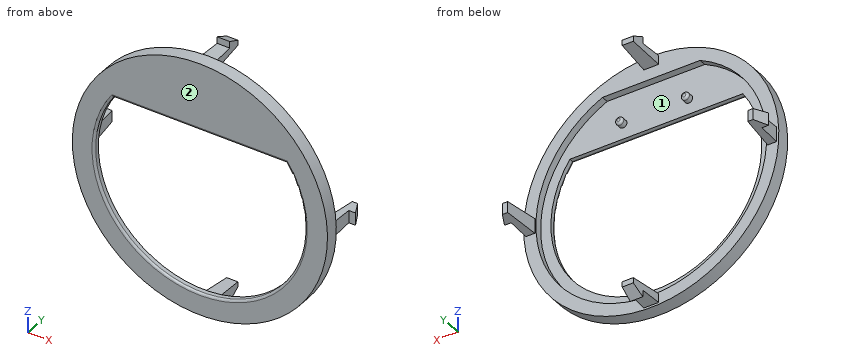
from build123d import *

# Parameters (mm, degrees)
SKETCH1_R           = 14.605
BOSS_EXTRUDE1_DEPTH = 1.524
CUT_EXTRUDE1_DEPTH  = 0.8128
SKETCH4_R           = 0.4445
BOSS_EXTRUDE2_DEPTH = 0.8128
CUT_EXTRUDE2_DEPTH  = 21.670575557
FILLET1_R           = 0.254
FILLET3_R           = 0.254
SNAP_START          = 13.7414
SNAP_HOOK1_DEPTH    = 0.6096
SNAP_START_2        = -0.714869456
SNAP_HOOK1_2_DEPTH  = 1.429738912
SNAP_START_3        = -0.847985215
SNAP_HOOK1_3_DEPTH  = 1.69597043
SNAP_START_4        = 12
SNAP_HOOK1_4_DEPTH  = 4
CIRPATTERN1_COUNT   = 4


with BuildPart() as part:
    # Sketch1 → Boss-Extrude1 (new body)
    with BuildSketch(Plane(origin=(0, 0, 0), x_dir=(1, 0, 0), z_dir=(0, 1, 0))):
        with Locations(Location((0, 0, 0), (0, 0, 270))):
            Circle(SKETCH1_R)
    extrude(amount=BOSS_EXTRUDE1_DEPTH)

    # Sketch3 → Cut-Extrude1 (cut)
    with BuildSketch(Plane(origin=(0, 1.524, 0), x_dir=(1, 0, 0), z_dir=(0, 1, 0))):
        with BuildLine():
            Line((-5.588, -11.967686493), (5.588, -11.967686493))
            ThreePointArc((5.588, -11.967686493), (0, 13.208), (-5.588, -11.967686493))
        make_face()
    extrude(amount=-CUT_EXTRUDE1_DEPTH, mode=Mode.SUBTRACT)

    # Sketch4 → Boss-Extrude2 (add)
    with BuildSketch(Plane(origin=(0, 0.7112, 0), x_dir=(1, 0, 0), z_dir=(0, 1, 0))):
        with Locations(Location((-3.7592, -8.6233, 0), (0, 0, 90))):
            Circle(SKETCH4_R)
        with Locations(Location((3.7592, -8.6233, 0), (0, 0, 90))):
            Circle(SKETCH4_R)
    extrude(amount=BOSS_EXTRUDE2_DEPTH)

    # Sketch5 → Cut-Extrude2 (cut, through all)
    with BuildSketch(Plane(origin=(0, 0.7112, 0), x_dir=(1, 0, 0), z_dir=(0, 1, 0))):
        with BuildLine():
            Line((-9.940854815, -6.887686493), (9.870656967, -6.887686493))
            ThreePointArc((9.870656967, -6.887686493), (-0.035098924, 12.065), (-9.940854815, -6.887686493))
        make_face()
    extrude(amount=-CUT_EXTRUDE2_DEPTH, mode=Mode.SUBTRACT)

    # Fillet1
    fillet1_edges = [part.edges().sort_by_distance(p)[0] for p in [
        (-0.035098924, 0, -12.065),
        (-0.035098924, 0, 6.887686493),
    ]]
    fillet(fillet1_edges, radius=FILLET1_R)

    # Fillet3
    fillet3_edges = [part.edges().sort_by_distance(p)[0] for p in [
        (-3.7592, 1.524, 9.0678),
        (3.7592, 1.524, 9.0678),
    ]]
    fillet(fillet3_edges, radius=FILLET3_R)

    # Snap Hook1: read off the stored shape, not the designer's step
    # Snap Hook1 outline → Snap Hook1 (add)
    with BuildSketch(Plane.XY.offset(SNAP_START)):
        Polygon((-0.847985215, 1.524), (0.847985215, 1.524), (0.635, 5.588), (-0.635, 5.588), align=None)
    snap_hook1 = extrude(amount=SNAP_HOOK1_DEPTH)

    # Snap Hook1 2 outline → Snap Hook1 2 (add)
    with BuildSketch(Plane.YZ.offset(SNAP_START_2)):
        Polygon((1.524, 13.7414), (1.524, 13.335), (5.588, 13.7414), align=None)
        Polygon((4.064, 15.113), (4.064, 14.351), (5.588, 14.351), align=None)
    snap_hook1_2 = extrude(amount=SNAP_HOOK1_2_DEPTH)

    # Snap Hook1 3 outline → Snap Hook1 3 (add)
    with BuildSketch(Plane.YZ.offset(SNAP_START_3)):
        Polygon((1.524, 13.7414), (1.524, 13.335), (5.588, 13.7414), align=None)
    snap_hook1_3 = extrude(amount=SNAP_HOOK1_3_DEPTH)

    # Snap Hook1 4 outline → Snap Hook1 4 (cut)
    with BuildSketch(Plane.XY.offset(SNAP_START_4)):
        Polygon((0.847985215, 1.524), (0.847985215, 7), (0.561000216, 7), (0.635, 5.588), align=None)
        Polygon((-0.635, 5.588), (-0.561000216, 7), (-0.847985215, 7), (-0.847985215, 1.524), align=None)
    snap_hook1_4 = extrude(amount=SNAP_HOOK1_4_DEPTH, mode=Mode.SUBTRACT)

    # CirPattern1: Snap Hook1, Snap Hook1 2, Snap Hook1 3, Snap Hook1 4 ×4 about axis
    cirpattern1_axis = Axis((0, 1.524, 0), (0, 1, 0))
    add([snap_hook1.rotate(cirpattern1_axis, i * 360 / CIRPATTERN1_COUNT) for i in range(1, CIRPATTERN1_COUNT)])
    add([snap_hook1_2.rotate(cirpattern1_axis, i * 360 / CIRPATTERN1_COUNT) for i in range(1, CIRPATTERN1_COUNT)])
    add([snap_hook1_3.rotate(cirpattern1_axis, i * 360 / CIRPATTERN1_COUNT) for i in range(1, CIRPATTERN1_COUNT)])
    add([snap_hook1_4.rotate(cirpattern1_axis, i * 360 / CIRPATTERN1_COUNT) for i in range(1, CIRPATTERN1_COUNT)], mode=Mode.SUBTRACT)


solid = part.part
CAD build for the part. Positions are in the model's coordinates, mm. Face numbers are marked on the shaded views. Round coordinates to 2 decimals unless told otherwise and drop trailing zeros. Order: outer loops, then holes, each group sorted by start corner. A loop starts at its lowest first (then second) coordinate and runs counter-clockwise, first axis right, second up. Notation, with made-up numbers: M 56.25,-18.5 L 100.25,-18.5 A23 ccw 100.25,5.5 Z; hole C 70,31.5 d10. An arc over 180 degrees is marked long. Use one line per item in the form item = value.
Q1. Probe L1, parallel to X at y = 1.25, z = 0 (3 decimals); L2, parallel to X at y = 0.5, z = 0 (3 decimals); L3, parallel to Y at x = 4.5, z = -13. List the from-to ranges inside material, lowest first.
Recorded:
L1 = -14.605 to -13.208, 13.208 to 14.605
L2 = -14.605 to -12.1, 12.03 to 14.605
L3 = 0 to 1.52
Q2. Saw through at B-B on z = 10. Give the cut face in (x, y), then the cut area to 3 significant figures.
Recorded:
outline = M -10.64,0 L 10.64,0 L 10.64,1.52 L 8.63,1.52 L 8.63,0.71 L -8.63,0.71 L -8.63,1.52 L -10.64,1.52 Z
area = 18.4 mm^2
Q3. Flat gauge pins, fed straight in: P1, Ø1.4, axis at x = 0.5, y = 3, coming from the -Z side; P2, Ø0.9, axis at x = -1, y = 1, coming from the -Z side; P3, Ø1.5, axis at x = -5, z = -11.5, coming from the +Y side; P4, Ø12, axis at x = 8.5, z = 6, coming from the -Y side. Where does each tip first touch, or does it go through?
Recorded:
P1 = -14.35
P2 = -14.59
P3 = 1.52
P4 = 0
Q4. Saw through at A-A on y = 4.9. Give the cut face in (x, z) (3 decimals).
Recorded:
outline = M -14.695,-0.671 L -13.673,-0.671 L -13.673,0.671 L -14.695,0.671 Z; M -0.671,-14.695 L 0.671,-14.695 L 0.671,-13.673 L -0.671,-13.673 Z; M -0.671,13.673 L 0.671,13.673 L 0.671,14.695 L -0.671,14.695 Z; M 13.673,-0.671 L 14.695,-0.671 L 14.695,0.671 L 13.673,0.671 Z
Q5. Two-plate mould, pull along X, no slides. Class the marked faces 1 and 2: +X half, -X half, draft (parallel to the pull), parting line (faces both ways), or undercut.
Recorded:
face_1 = undercut
face_2 = draft
